The listing builds one solid part. Answer for the finished solid, in the listing's coordinates (mm). A direction names the side the tool comes from. Coordinates: 2 decimals unless noted, no trailing zeros. Write each loop counter-clockwise with the first axis right and the second up, starting at its lowest first coordinate (ties: lowest second). Pieces come first, ordered by that corner, then holes.
(1) For a pull along X with two mould halves and no side action, classify faces 1 (the flat face through (-36.908, 129.179, 2.465)), 2 (the flat face through (65, 77, 3)), 3 (the flat face through (66.03, 129.89, 2.46)) as +X half, -X half, draft (parallel to the pull), parting line (faces both ways), or undercut.
(2) Given P1, Ø2.5, axis at y = 78, z = 2, coming from the +X side, flat-ended and moving along its own axis, determine where the tip first touches the part or whether it passes through.
(3) The part is cut by section B-B on z = 0.75. Determine the outline of the cut face in (x, y), plus the area to 3 significant figures.
(4) Straight lines are drawn through the part: line 1 (X direction, y = 79.5, z = 1.9); line 2 (Y direction, x = 54.5, z = 3.1) (1 decimal); line 3 (Y direction, x = 50, z = 2.1) (3 decimals). For each, find the intervals that lie inside material, in ascending order.
(5) The part is cut by section D-D on x = 67. Determine the outline of the cut face in (y, z), plus the area to 3 significant figures.
(6) The part is cut by section C-C on y = 90. Determine the outline of the cut face in (x, z), plus the area to 3 significant figures.
(7) The part is cut by section A-A on x = 22.5. Determine the outline of the cut face in (y, z).
(8) Which of the six approach directions +Z, -Z, +X, -X, +Y, -Y give full straight-line access (tool end or side, diameter ignored) to faces 4 (the cylindrical face through (44.397, 1.253, 2.535)), 5 (the flat face through (37, 80, 3)), 6 (the flat face through (-32.255, 40.018, 2.465))?
from build123d import *

# Parameters (mm, degrees)
GRUNDPLATTE_DEPTH      = 5
SKIZZE2_W              = 55
SKIZZE2_H              = 5
NUTH_HENLEITWERK_DEPTH = 15
VERRUNDUNG1_R          = 10
VERRUNDUNG2_R          = 3


with BuildPart() as part:
    # Skizze1 → Grundplatte (new body)
    with BuildSketch(Plane.XY):
        Polygon((-50, 186), (35, 186), (95, 77.5), (45, 0), (0, 0), (-40, 0), (-25, 77.5), align=None)
    extrude(amount=GRUNDPLATTE_DEPTH)

    # Skizze2 → NutHöhenleitwerk (cut)
    with BuildSketch(Plane.XY.offset(5)):
        with Locations((37.5, 77.5)):
            Rectangle(SKIZZE2_W, SKIZZE2_H)
    extrude(amount=-NUTH_HENLEITWERK_DEPTH, mode=Mode.SUBTRACT)

    # Verrundung1
    verrundung1_edges = [part.edges().sort_by_distance(p)[0] for p in [
        (35, 186, 2.5),
        (45, 0, 2.5),
    ]]
    fillet(verrundung1_edges, radius=VERRUNDUNG1_R)

    # Verrundung2
    verrundung2_edges = [part.edges().sort_by_distance(p)[0] for p in [
        (-50, 186, 2.5),
        (-40, 0, 2.5),
    ]]
    fillet(verrundung2_edges, radius=VERRUNDUNG2_R)


solid = part.part
Model answer:
1. face 1: -X half
1. face 2: undercut
1. face 3: +X half
2. P1: stops at x = 95
3. outline: (-49.15, 182.33) - (-25, 77.5) - (-39.31, 3.57) arc R3 ccw to (-36.36, 0) - (39.55, 0) arc R10 ccw to (47.95, 4.58) - (95, 77.5) - (37.85, 180.84) arc R10 ccw to (29.1, 186) - (-46.23, 186) arc R3 ccw to start; hole (10, 75) - (65, 75) - (65, 80) - (10, 80) - close
3. area: 18,800 mm2
4. line 1: x = -25.46 to 10, 65 to 93.89
4. line 2: y = 14.7 to 75, 80 to 150.7
4. line 3: y = 7.75 to 75, 80 to 158.875
5. outline: (34.1, 0) - (128.13, 0) - (128.13, 5) - (34.1, 5) - close
5. area: 470 mm2
6. outline: (-27.88, 0) - (88.09, 0) - (88.09, 5) - (-27.88, 5) - close
6. area: 580 mm2
7. outline: (0, 0) - (75, 0) - (75, 5) - (0, 5) - close; (80, 0) - (186, 0) - (186, 5) - (80, 5) - close
8. face 4: +Z, -Z, +X, -Y
8. face 5: +Z, -Z
8. face 6: +Z, -Z, -X
